The model under review builds one solid part; all positions refer to its coordinate system, in mm. A direction names the side the tool comes from. Round coordinates to 2 decimals unless told otherwise and drop trailing zeros. Order: outer loops, then holes, each group sorted by start corner. A loop starts at its lowest first (then second) coordinate and runs counter-clockwise, first axis right, second up. Notation, with made-up numbers: M 43.25,89 L 56.25,89 A25 ccw 56.25,103 Z; hole C -19.75,17.5 d8. An arc over 180 degrees is marked long. One line per item, written item: value. Start each with the question number.
Autodesk Inventor part; units mm, degrees
ref_plane "YZ Plane" through (0, 0, 0) normal (1, 0, 0) x (0, 1, 0)
ref_plane "XZ Plane" through (0, 0, 0) normal (0, 1, 0) x (-1, 0, 0)
ref_plane "XY Plane" through (0, 0, 0) normal (0, 0, 1) x (1, 0, 0)
sketch "Sketch1" plane through (0, 0, 0) normal (1, 0, 0) x (0, 1, 0)
  line L0 (3.175, 0) -> (53.975, 0)
  line L1 (57.15, 3.175) -> (57.15, 53.975)
  line L2 (53.975, 57.15) -> (3.175, 57.15)
  line L3 (0, 53.975) -> (0, 3.175)
  arc A0 (3.175, 57.15) -> (0, 53.975) centre (3.175, 53.975) ccw
  arc A1 (57.15, 53.975) -> (53.975, 57.15) centre (53.975, 53.975) ccw
  arc A2 (53.975, 0) -> (57.15, 3.175) centre (53.975, 3.175) ccw
  arc A3 (0, 3.175) -> (3.175, 0) centre (3.175, 3.175) ccw
  point P0 (0, 0)
  point P1 (57.15, 57.15)
  point P2 (57.15, 0)
  point P3 (0, 57.15)
  dimension "d0" = 57.15
  dimension "d1" = 57.15
  dimension "d17" = 3.175
extrude "Extrusion1" add sketch "Sketch1" along normal blind 78.74
sketch "Sketch2" plane through (0, 0, 0) normal (-1, 0, 0) x (0, 0, 1)
  line L0 (0, 53.975) -> (0, 3.175)
  line L1 (53.975, 57.15) -> (3.175, 57.15)
  circle A0 centre (28.575, 28.575) radius 19.05
  point P0 (0, 57.15)
  point P1 (0, 0)
  point P2 (57.15, 57.15)
  dimension "d4" = 38.1
  dimension "d18" = 28.575
  dimension "d19" = 28.575
extrude "Extrusion2" add sketch "Sketch2" along normal blind 1.524
sketch "Sketch3" plane through (-1.524, 28.575, 28.575) normal (-1, 0, 0) x (0, 0, 1)
  circle A0 centre (0, 0) radius 19.05
  circle A1 centre (0, 0) radius 3.175
  point P0 (-28.575, -28.575)
  dimension "d10" = 6.35
extrude "Extrusion3" add sketch "Sketch3" along normal blind 19.05 contours A1
sketch "Sketch4" plane through (-20.574, 28.575, 28.575) normal (-1, 0, 0) x (0, 0, 1)
  circle A0 centre (0, 0) radius 3.175
  line L0 (-1.7227, 2.667) -> (1.7227, 2.667)
  line L1 (0, -3.175) -> (-5.2914, -3.175)
  point P0 (-28.575, -28.575)
  dimension "d13" = 5.842
extrude "Extrusion4" cut sketch "Sketch4" against normal blind 14.986 contours L0 A0 picked at (-0.1211, 2.8294)
sketch "Sketch5" plane through (78.74, 0, 0) normal (1, 0, 0) x (0, 0, -1)
  line L0 (-57.15, 53.975) -> (-57.15, 3.175)
  arc A0 (-57.15, 3.175) -> (-53.975, 0) centre (-53.975, 3.175) ccw
  line L1 (-53.975, 0) -> (-3.175, 0)
  arc A1 (-3.175, 0) -> (0, 3.175) centre (-3.175, 3.175) ccw
  line L2 (0, 3.175) -> (0, 53.975)
  arc A2 (0, 53.975) -> (-3.175, 57.15) centre (-3.175, 53.975) ccw
  line L3 (-3.175, 57.15) -> (-53.975, 57.15)
  arc A3 (-53.975, 57.15) -> (-57.15, 53.975) centre (-53.975, 53.975) ccw
  circle A4 centre (-52.197, 52.197) radius 2.54
  circle A5 centre (-52.197, 52.197) radius 4.953
  line L4 (-3.175, 57.15) -> (-53.975, 57.15)
  line L5 (-52.197, 47.244) -> (-57.15, 47.244)
  line L6 (-57.15, 47.244) -> (-57.15, 57.15)
  line L7 (-57.15, 57.15) -> (-47.244, 57.15)
  line L8 (-47.244, 57.15) -> (-47.244, 52.197)
  circle A6 centre (-4.953, 52.197) radius 4.953
  circle A7 centre (-4.953, 4.953) radius 4.953
  circle A8 centre (-52.197, 4.953) radius 4.953
  line L9 (0, 3.175) -> (0, 53.975)
  line L10 (-53.975, 0) -> (-3.175, 0)
  line L11 (-57.15, 53.975) -> (-57.15, 3.175)
  line L12 (0, 57.15) -> (-9.906, 57.15)
  line L13 (-9.906, 57.15) -> (-9.906, 52.197)
  line L14 (-4.953, 47.244) -> (0, 47.244)
  line L15 (0, 47.244) -> (0, 57.15)
  line L16 (-57.15, 0) -> (-47.244, 0)
  line L17 (-47.244, 0) -> (-47.244, 4.953)
  line L18 (-52.197, 9.906) -> (-57.15, 9.906)
  line L19 (-57.15, 9.906) -> (-57.15, 0)
  line L20 (-4.953, 9.906) -> (0, 9.906)
  line L21 (0, 9.906) -> (0, 0)
  line L22 (0, 0) -> (-9.906, 0)
  line L23 (-9.906, 0) -> (-9.906, 4.953)
  dimension "d48" = 4.953
  dimension "d49" = 4.953
  dimension "d50" = 5.08
  dimension "d51" = 9.906
  dimension "d52" = 9.906
  dimension "d53" = 9.906
  dimension "d54" = 9.906
  dimension "d55" = 9.906
  dimension "d56" = 9.906
  dimension "d57" = 9.906
  dimension "d58" = 9.906
  dimension "d59" = 9.906
  dimension "d60" = 9.906
  dimension "d61" = 9.906
  dimension "d62" = 9.906
  dimension "d63" = 9.906
extrude "Extrusion6" cut sketch "Sketch5" against normal blind 74.041 contours L0 A5 L5 | L18 A8 L0 | L0 A3 L3 A5 | A5 | A8 L1 A0 L0 | A8 | L6 L7 A3 | L3 L8 A5 | A0 L16 L19 | A8 L17 L1 | L3 A6 L13 | L23 A7 L1 | L3 A2 L2 A6 | A6 | A7 L2 A1 L1 | A7 | L12 L15 A2 | L2 L14 A6 | A1 L21 L22 | A7 L20 L2 | A4
fillet "Fillet1" radius 1.905 8 edges at (41.7195, 57.15, 47.244) (41.7195, 47.244, 57.15) (41.7195, 57.15, 9.906) (41.7195, 47.244, 0) (41.7195, 9.906, 0) (41.7195, 0, 9.906) (41.7195, 0, 47.244) (41.7195, 9.906, 57.15)
sketch "Sketch6" plane through (0, 0, 0) normal (-1, 0, 0) x (0, 0, 1)
  line L0 (53.975, 57.15) -> (3.175, 57.15)
  line L1 (0, 53.975) -> (0, 3.175)
  point P0 (0, 0)
  point P1 (4.953, 52.197)
  point P2 (52.197, 52.197)
  point P3 (52.197, 4.953)
  point P4 (4.953, 4.953)
  dimension "d36" = 47.244
  dimension "d37" = 47.244
  dimension "d39" = 4.953
  dimension "d40" = 4.953
hole "Hole1" at (0, 52.197, 4.953) at (0, 52.197, 52.197) at (0, 4.953, 52.197) at (0, 4.953, 4.953) direction (1, 0, 0) diameter 5.08 end through all
properties part number "G723-280-4"
Item 1: Clearance check with flat-ended pins moving along their axes: P1, Ø1.5, axis at x = 25.5, z = 53.5, coming from the +Y side; P2, Ø8, axis at y = 27.5, z = 39, coming from the -X side; P3, Ø8, axis at y = 52.197, z = 52.197, coming from the +X side; P4, Ø11.5, axis at y = 21, z = 24.5, coming from the -X side. State where each tip first meets the part, or that it passes through.
Item 2: Consider section D-D, the plane y = 33.5. Give the boundary of the cut face in (x, z).
Item 3: The part is to be moulded in two halves that separate along Z. For faces 1 (the flat face through (39, 28, 0)), 2 (the flat face through (4.699, 53, 2)), 3 (the cylindrical face through (2.38, 49.68, 4.62)), say which applies: pulls with the +Z half, pulls with the -Z half, needs draft (parallel to the pull), parting line crosses it, or undercut.
Item 4: Wall thickness on L1, parallel to Y at x = 68, z = 45.5; L2, parallel to X at y = 35, z = 31; L3, parallel to Y at x = 21.5, z = 52.5: over which ranges is each line inside the solid? List them lowest first.
Item 5: Consider section C-C, the plane z = 43.5. Give the boundary of the cut face in (x, y).
Item 6: Consider section A-A, the plane x = 24. Give the boundary of the cut face in (y, z) (3 decimals).
Item 7: Consider section B-B, the plane y = 51. Give the boundary of the cut face in (x, z), then the cut area to 3 significant figures.
Item 8: Machinability: for faces 4 (the flat face through (4.699, 5, 2)), 5 (the flat face through (4.699, 50, 54)), 6 (the cylindrical face through (-10.916, 25.427, 28.162)), which of the approach directions +Z, -Z, +X, -X, +Y, -Y give a long, thin tool a straight path to every point of the face, cutting with its end or side? Answer none if there is none.
Computed:
1. P1: stops at y = 47.24
1. P2: stops at x = -1.52
1. P3: stops at x = 4.7
1. P4: stops at x = -20.57
2. outline: M -1.52,10.17 L 0,10.17 L 0,0 L 78.74,0 L 78.74,57.15 L 0,57.15 L 0,46.98 L -1.52,46.98 Z
3. face 1: pulls with the -Z half
3. face 2: needs draft
3. face 3: undercut
4. L1: y = 0.01 to 57.14
4. L2: x = -1.52 to 78.74
4. L3: y = 9.91 to 47.24
5. outline: M -1.52,16.74 L 0,16.74 L 0,0 L 78.74,0 L 78.74,57.15 L 0,57.15 L 0,40.41 L -1.52,40.41 Z
6. outline: M 0,11.811 A1.905 ccw 1.905,9.906 L 4.953,9.906 A4.953 cw 9.906,4.953 L 9.906,1.905 A1.905 ccw 11.811,0 L 45.339,0 A1.905 ccw 47.244,1.905 L 47.244,4.953 A4.953 cw 52.197,9.906 L 55.245,9.906 A1.905 ccw 57.15,11.811 L 57.15,45.339 A1.905 ccw 55.245,47.244 L 52.197,47.244 A4.953 cw 47.244,52.197 L 47.244,55.245 A1.905 ccw 45.339,57.15 L 11.811,57.15 A1.905 ccw 9.906,55.245 L 9.906,52.197 A4.953 cw 4.953,47.244 L 1.905,47.244 A1.905 ccw 0,45.339 Z
7. outline: M 0,0 L 4.7,0 L 4.7,2.71 L 0,2.71 Z; M 0,7.19 L 4.7,7.19 L 4.7,9.76 L 78.74,9.76 L 78.74,47.39 L 4.7,47.39 L 4.7,49.96 L 0,49.96 Z; M 0,54.44 L 4.7,54.44 L 4.7,57.15 L 0,57.15 Z
7. area: 3,010 mm^2
8. face 4: -Z, +X, -Y
8. face 5: +Z, +X, +Y
8. face 6: -X
